```python
from build123d import *

# Parameters (mm, degrees)
F0_R     = 11.5
F0_R_2   = 1.05
F0_R_3   = 1
F1_DEPTH = 5


with BuildPart() as f1:
    # F0 (on Right) → F1 (new body)
    with BuildSketch(Plane.YZ):
        Circle(F0_R)
        with Locations((0, -9)):
            Circle(F0_R_2, mode=Mode.SUBTRACT)
        with Locations((-9, 0)):
            Circle(F0_R_3, mode=Mode.SUBTRACT)
        with BuildLine():
            ThreePointArc((-5.65, 3.65), (-5.064214, 5.064214), (-3.65, 5.65))
            Line((-3.65, 5.65), (3.65, 5.65))
            ThreePointArc((3.65, 5.65), (5.064214, 5.064214), (5.65, 3.65))
            Line((5.65, 3.65), (5.65, -3.65))
            ThreePointArc((5.65, -3.65), (5.064214, -5.064214), (3.65, -5.65))
            Line((3.65, -5.65), (-3.65, -5.65))
            ThreePointArc((-3.65, -5.65), (-5.064214, -5.064214), (-5.65, -3.65))
            Line((-5.65, -3.65), (-5.65, 3.65))
        make_face(mode=Mode.SUBTRACT)
        with Locations((9, 0)):
            Circle(F0_R_3, mode=Mode.SUBTRACT)
        with Locations((0, 9)):
            Circle(F0_R_2, mode=Mode.SUBTRACT)
    extrude(amount=F1_DEPTH)

    # F3 (on offset) → F5 (revolve, cut)
    with BuildSketch(Plane.XZ.offset(9)):
        Polygon((2.3, 0), (5, 0), (5, 2.2), (4.5, 2.2), align=None)
    revolve(axis=Axis((2.750115, -9, 0), (1, 0, 0)), mode=Mode.SUBTRACT)

    # F7 (on offset) → F8 (revolve, cut)
    with BuildSketch(Plane.XZ.offset(-9)):
        Polygon((4.5, 2.2), (2.3, 0), (5, 0), (5, 2.2), align=None)
    revolve(axis=Axis((3.65, 9, 0), (1, 0, 0)), mode=Mode.SUBTRACT)


solid = f1.part
```
For this review, take the finished solid that the model builds, in its own axes (mm). A direction names the side the tool comes from. Coordinates: 2 decimals unless noted, no trailing zeros. Write each loop counter-clockwise with the first axis right and the second up, starting at its lowest first coordinate (ties: lowest second). Pieces come first, ordered by that corner, then holes. Notation, with made-up numbers: (83, 56.5) - (107, 56.5) arc R13 cw to (107, 65.5) - close; hole circle Ø9 at (-23, 10). An arc over 180 degrees is marked (long way). Answer in a Markdown table with one row per item. Add a question column.
Q1. We need section A-A, the plane y = 0. State the section outline as (x, z) points.
Q2. We need section D-D, the plane z = -9. State the section outline as (x, y) points.
Q3. Draft analysis for pull direction Z (two halves, no side actions). For faces 4 (the cylindrical face through (2.5, -1.5, 11.4)), 5 (the cylindrical face through (2.46, 0.56, 9.89)), 6 (the flat face through (5, -0.2, -7.5)), state which applies: +Z half, -Z half, draft (parallel to the pull), parting line (faces both ways), or undercut.
Q4. For probe 1 along Z at (x, y) = (2.25, 0); probe 2 along Z at (x, y) = (1.2, -0.75); probe 3 along Y at (x, z) = (1.8, -0.25), list the stretches that pass through material, from the lowest coordinate up.
Q5. Tool access review of faces 1 (the flat face through (2, 5.65, 0)), 2 (the flat face through (0, 7.5, 0.2)), 3 (the cylindrical face through (4.746, -10.855, 1.183)): name each direction out of +Z, -Z, +X, -X, +Y, -Y from which nothing blocks a thin tool from reaching the whole face with its end or side.
Q6. For P1, Ø1.6, axis at y = -9, z = 0, coming from the +X side; P2, Ø1, axis at x = 1, y = 7.5, coming from the +Z side, all flat-tipped, find the tip position at first contact; note any pin that passes through.
Q7. We need section B-B, the plane z = 0. State the section outline as (x, y) points.
Q8. We need section C-C, the plane x = 0.95. State the section outline as (y, z) points.
Answer list:
| question | item | result |
|---|---|---|
| 1 | outline | (0, -11.5) - (5, -11.5) - (5, -10.05) - (0, -10.05) - close; (0, -7.95) - (5, -7.95) - (5, -5.65) - (0, -5.65) - close; (0, 5.65) - (5, 5.65) - (5, 7.95) - (0, 7.95) - close; (0, 10.05) - (5, 10.05) - (5, 11.5) - (0, 11.5) - close |
| 2 | outline | (0, -7.16) - (5, -7.16) - (5, -1.05) - (0, -1.05) - close; (0, 1.05) - (5, 1.05) - (5, 7.16) - (0, 7.16) - close |
| 3 | face 4 | parting line |
| 3 | face 5 | undercut |
| 3 | face 6 | draft |
| 4 | probe 1 | z = -11.5 to -10.05, -7.95 to -5.65, 5.65 to 7.95, 10.05 to 11.5 |
| 4 | probe 2 | z = -11.48 to -9.73, -8.27 to -5.65, 5.65 to 8.27, 9.73 to 11.48 |
| 4 | probe 3 | y = -11.5 to -9.97, -8.03 to -5.65, 5.65 to 8.03, 9.97 to 11.5 |
| 5 | face 1 | +X, -X |
| 5 | face 2 | +Z, -Z, -X, +Y, -Y |
| 5 | face 3 | +X |
| 6 | P1 | passes through |
| 6 | P2 | stops at z = 9.12 |
| 7 | outline | (0, -11.5) - (5, -11.5) - (5, -11.2) - (4.5, -11.2) - (3.3, -10) - (0, -10) - close; (0, -8) - (3.3, -8) - (4.5, -6.8) - (5, -6.8) - (5, -5.65) - (0, -5.65) - close; (0, 5.65) - (5, 5.65) - (5, 6.8) - (4.5, 6.8) - (3.3, 8) - (0, 8) - close; (0, 10) - (3.3, 10) - (4.5, 11.2) - (5, 11.2) - (5, 11.5) - (0, 11.5) - close |
| 8 | outline | circle Ø23 at (0, 0); hole circle Ø2 at (-9, 0); hole (-5.65, -3.65) arc R2 ccw to (-3.65, -5.65) - (3.65, -5.65) arc R2 ccw to (5.65, -3.65) - (5.65, 3.65) arc R2 ccw to (3.65, 5.65) - (-3.65, 5.65) arc R2 ccw to (-5.65, 3.65) - close; hole circle Ø2.1 at (0, -9); hole circle Ø2.1 at (0, 9); hole circle Ø2 at (9, 0) |
